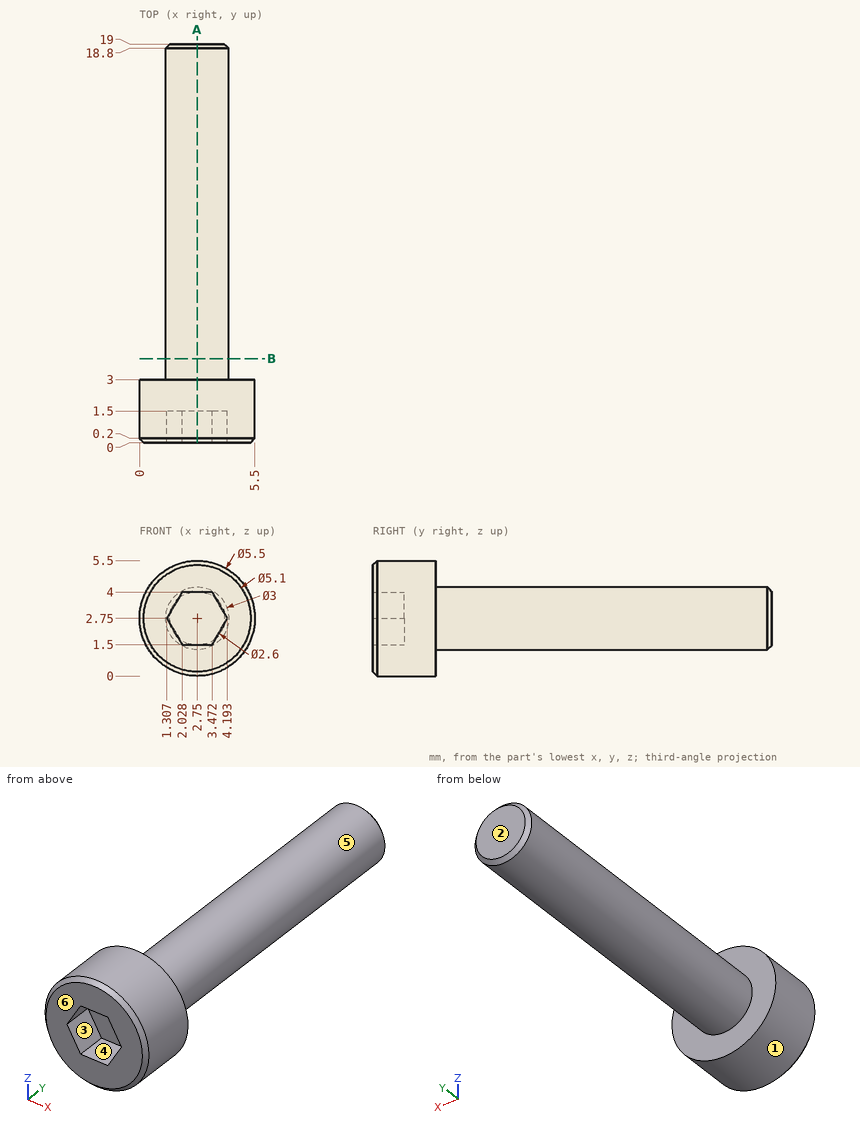
Study the drawing (mm; zero at the part's minimum x, y, z) and answer. A direction names the side the tool comes from. Round coordinates to 2 decimals unless told otherwise and drop trailing zeros. Write each loop counter-clockwise with the first axis right and the second up, starting at its lowest first coordinate (ties: lowest second). Pieces come first, ordered by that corner, then holes.
1) Which of the six approach directions +Z, -Z, +X, -X, +Y, -Y give full straight-line access (tool end or side, diameter ignored) to the marked faces 4, 5 and 6?
2) Consider probe 1 along X at (y, z) = (17.5, 3.15) (1 decimal); probe 2 along Z at (x, y) = (3.95, 1.25) (1 decimal); probe 3 along Y at (x, z) = (4.4, 2.25). Determine where each line is inside the solid, lowest interval first.
3) Determine the mould class of the marked faces 1, 2 and 3 for opening direction X: pulls with the +X half, pulls with the -X half, needs draft (parallel to the pull), parting line crosses it, or undercut.
4) Flat-ended cylindrical pins translate along their axes: P1, Ø2, axis at y = 9, z = 3.5, coming from the +X side; P2, Ø3, axis at y = 15, z = 1, coming from the -X side; P3, Ø1, axis at x = 4.5, z = 4, coming from the +Y side. Find the tip coordinate at first contact, or state that the pin passes through.
5) A cutting plane is placed at B-B on y = 4. Determine the outline of the cut face in (x, z).
6) A cutting plane is placed at A-A on x = 2.75. Determine the outline of the cut face in (y, z).
Entries:
1. face 4: -Y
1. face 5: +Y
1. face 6: +Z, -Z, +X, -X, -Y
2. probe 1: x = 1.3 to 4.2
2. probe 2: z = 0.3 to 2.3, 3.2 to 5.2
2. probe 3: y = 0 to 3
3. face 1: parting line crosses it
3. face 2: needs draft
3. face 3: undercut
4. P1: stops at x = 4.25
4. P2: stops at x = 1.27
4. P3: stops at y = 3
5. outline: circle Ø3 at (2.75, 2.75)
6. outline: (0, 0.2) - (0.2, 0) - (3, 0) - (3, 1.25) - (18.8, 1.25) - (19, 1.45) - (19, 4.05) - (18.8, 4.25) - (3, 4.25) - (3, 5.5) - (0.2, 5.5) - (0, 5.3) - (0, 4) - (1.5, 4) - (1.5, 1.5) - (0, 1.5) - close
